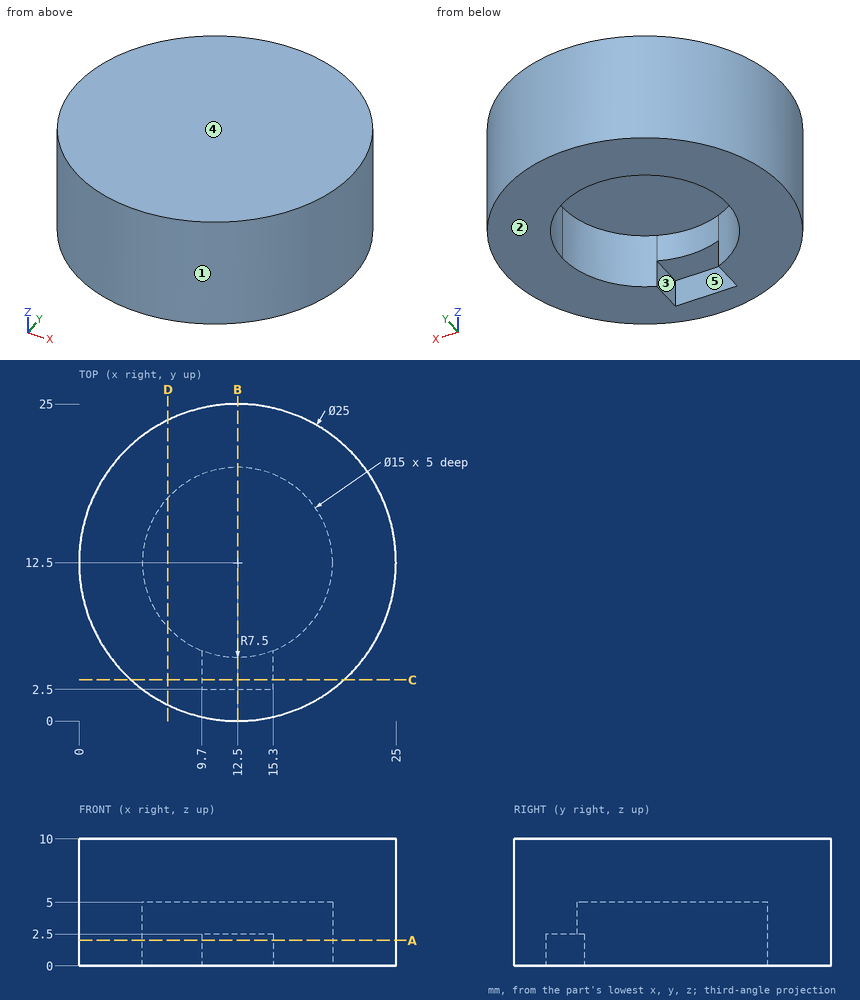
Geometry: see drawing. Coordinates: mm, zero at the bounding-box minimum. A direction names the side the tool comes from. Round coordinates to 2 decimals unless told otherwise and drop trailing zeros. Loops run counter-clockwise (first coordinate to the right, second up) from the corner with the lowest first, then second, coordinate; pieces in that order, holes last. Notation, with made-up numbers: M 51.25,40 L 59.25,40 A15 cw 59.25,65 Z; hole C 48,29 d6. An arc over 180 degrees is marked long. Use a Markdown table: item, result. Add a question column.
1. Cut plane C-C, the plane y = 3.25. Output: boundary loops of the cut face in (x, z).
2. Pull-direction query (Y, two-part tool) for the marked faces 1, 2 and 3; classes: +Y half, -Y half, draft (parallel to the pull), parting line (faces both ways), or undercut.
3. Cut plane A-A, the plane z = 2. Output: boundary loops of the cut face in (x, y).
4. Ray query, line 1 along Y through (x, z) = (12.5, 2.45); line 2 along Y through (x, z) = (12.5, 3.15); line 3 along Z through (x, y) = (13.25, 7). Return the intervals inside material, ascending. Write a range as [from, to].
5. Cut plane B-B, the plane x = 12.5. Output: boundary loops of the cut face in (y, z).
6. Contact query for flat-ended pins moving along their axis: pin 1 (12 mm diameter, centred on x = 12.5, y = 12.5, fed in from -Z); pin 2 (4 mm diameter, centred on x = 15, z = 7, fed in from +Y); pin 3 (0.8 mm diameter, centred on y = 3.5, z = 1.5, fed in from +X). Output: stop coordinate, or through.
7. Cut plane D-D, the plane x = 7. Output: boundary loops of the cut face in (y, z).
8. Set-up query: the marked faces 4 and 5. Return all of +Z, -Z, +X, -X, +Y, -Y with unobstructed straight access to the full face (end or side cutting, diameter ignored); none if empty.
Solution:
| question | item | result |
|---|---|---|
| 1 | outline | M 4.09,0 L 9.7,0 L 9.7,2.5 L 15.3,2.5 L 15.3,0 L 20.91,0 L 20.91,10 L 4.09,10 Z |
| 2 | face 1 | parting line |
| 2 | face 2 | draft |
| 2 | face 3 | undercut |
| 3 | outline | C 12.5,12.5 d25; hole M 9.7,2.5 L 15.3,2.5 L 15.3,5.54 A7.5 ccw long 9.7,5.54 Z |
| 4 | line 1 | y = [0, 2.5], [20, 25] |
| 4 | line 2 | y = [0, 5], [20, 25] |
| 4 | line 3 | z = [5, 10] |
| 5 | outline | M 0,0 L 2.5,0 L 2.5,2.5 L 5,2.5 L 5,5 L 20,5 L 20,0 L 25,0 L 25,10 L 0,10 Z |
| 6 | pin 1 | stops at z = 5 |
| 6 | pin 2 | stops at y = 24.99 |
| 6 | pin 3 | stops at x = 21.57 |
| 7 | outline | M 1.28,0 L 7.4,0 L 7.4,5 L 17.6,5 L 17.6,0 L 23.72,0 L 23.72,10 L 1.28,10 Z |
| 8 | face 4 | +Z, +X, -X, +Y, -Y |
| 8 | face 5 | -Z |
